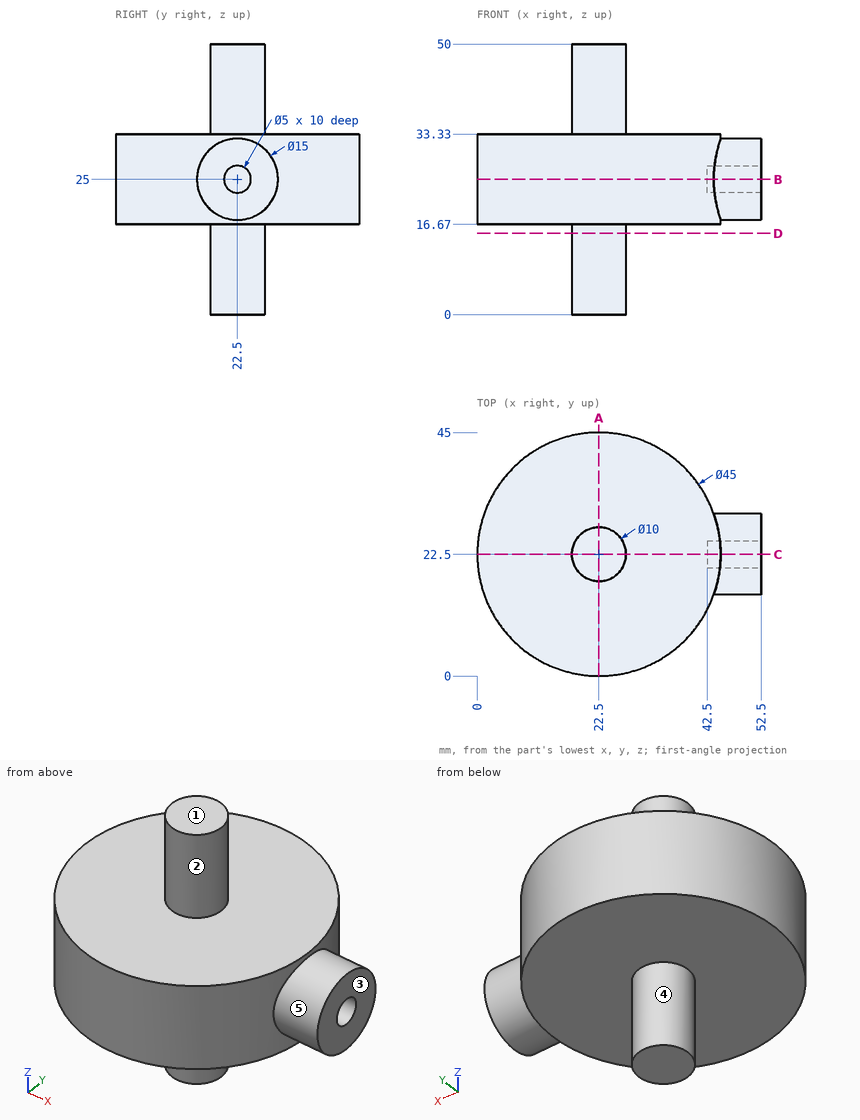
Input: dimensioned drawing with shaded views. Units: mm. Origin: part minimum x, y, z. A direction names the side the tool comes from. Coordinates: 2 decimals unless noted, no trailing zeros. Order: outer loops, then holes, each group sorted by start corner. A loop starts at its lowest first (then second) coordinate and runs counter-clockwise, first axis right, second up. Notation, with made-up numbers: (19.5, 27.5) - (63.5, 27.5) arc R25 ccw to (63.5, 51.5) - close; hole circle Ø5 at (68, -10.75). An arc over 180 degrees is marked (long way). One line per item, written item: value.
1) Cut plane D-D on z = 15. Output: boundary loops of the cut face in (x, y).
Computed values:
outline: circle Ø10 at (22.5, 22.5)
2) Cut plane C-C on y = 22.5. Output: boundary loops of the cut face in (x, z).
Computed values:
outline: (0, 16.67) - (17.5, 16.67) - (17.5, 0) - (27.5, 0) - (27.5, 16.67) - (45, 16.67) - (45, 17.5) - (52.5, 17.5) - (52.5, 22.5) - (42.5, 22.5) - (42.5, 27.5) - (52.5, 27.5) - (52.5, 32.5) - (45, 32.5) - (45, 33.33) - (27.5, 33.33) - (27.5, 50) - (17.5, 50) - (17.5, 33.33) - (0, 33.33) - close
3) Cut plane B-B on z = 25. Output: boundary loops of the cut face in (x, y).
Computed values:
outline: (42.5, 20) - (42.5, 25) - (52.5, 25) - (52.5, 30) - (43.71, 30) arc R22.5 ccw (long way) to (43.71, 15) - (52.5, 15) - (52.5, 20) - close
4) Contact query for flat-ended pins moving along their axis: pin 1 (8 mm diameter, centred on x = 43.5, y = 10, fed in from +Z); pin 2 (5 mm diameter, centred on y = 17, z = 6.5, fed in from -X); pin 3 (12 mm diameter, centred on x = 45.5, y = 32.5, fed in from -Z). Output: stop coordinate, or through.
Computed values:
pin 1: stops at z = 33.33
pin 2: stops at x = 18.5
pin 3: stops at z = 16.67
5) Ray query, line 1 (Y direction, x = 47, z = 25); line 2 (Z direction, x = 16, y = 4.5); line 3 (Z direction, x = 48, y = 22). Return the intervals inside material, ascending. Write a range as [from, to].
Computed values:
line 1: y = [15, 20], [25, 30]
line 2: z = [16.67, 33.33]
line 3: z = [17.52, 22.55], [27.45, 32.48]
6) Cut plane A-A on x = 22.5. Output: boundary loops of the cut face in (y, z), plus the area to 3 significant figures.
Computed values:
outline: (0, 16.67) - (17.5, 16.67) - (17.5, 0) - (27.5, 0) - (27.5, 16.67) - (45, 16.67) - (45, 33.33) - (27.5, 33.33) - (27.5, 50) - (17.5, 50) - (17.5, 33.33) - (0, 33.33) - close
area: 1,080 mm^2
7) Reachability of the marked faces 1, 2, 3, 4 and 5 from +Z, -Z, +X, -X, +Y, -Y: full face, straight path, thin tool, end or side. Return the list, or none.
Computed values:
face 1: +Z, +X, -X, +Y, -Y
face 2: +Z
face 3: +Z, -Z, +X, +Y, -Y
face 4: -Z
face 5: +X
